from build123d import *

# Parameters (mm, degrees)
F0_R     = 59
F0_R_2   = 49
F1_DEPTH = 3
F0_R_3   = 45
F2_DEPTH = 15
F3_SIZE  = 3


with BuildPart() as f1:
    # F0 (on Top) → F1 (new body)
    with BuildSketch(Plane.XY):
        with Locations((-35.217796, 30.469857)):
            Circle(F0_R)
        with Locations((-35.217796, 30.469857)):
            Circle(F0_R_2, mode=Mode.SUBTRACT)
    extrude(amount=F1_DEPTH)

    # F0 (on Top) → F2 (join)
    with BuildSketch(Plane.XY):
        with Locations((-35.217796, 30.469857)):
            Circle(F0_R_2)
        with Locations((-35.217796, 30.469857)):
            Circle(F0_R_3, mode=Mode.SUBTRACT)
    extrude(amount=F2_DEPTH)

    # F3
    f3_edges = [f1.edges().sort_by_distance(p)[0] for p in [
        (-80.217796, 30.469857, 15),
    ]]
    chamfer(f3_edges, length=F3_SIZE)


solid = f1.part
The model under review builds one solid part; all positions refer to its coordinate system, in mm. A direction names the side the tool comes from. Round coordinates to 2 decimals unless told otherwise and drop trailing zeros. Write each loop counter-clockwise with the first axis right and the second up, starting at its lowest first coordinate (ties: lowest second). Pieces come first, ordered by that corner, then holes. Notation, with made-up numbers: (-2, 5) - (10, 5) arc R29 cw to (10, 41) - close; hole circle Ø9 at (87.25, 22.5). An arc over 180 degrees is marked (long way). One line per item, written item: value. Start each with the question number.
1. Clearance check with flat-ended pins moving along their axes: P1, Ø1, axis at x = -74, z = 9, coming from the +Y side; P2, Ø6, axis at y = 22.5, z = 12, coming from the +X side; P3, Ø8, axis at y = -9.5, z = 2, coming from the +X side. State where each tip first meets the part, or that it passes through.
2. Consider section A-A on z = 13.5. Write out the cut boundary in (x, y).
3. The part is to be moulded in two halves that separate along Y. For faces 1 (the face through (-41.076, 75.087, 5.916)), 2 (the face through (-71.33, 63.59, 8.92)), 3 (the face through (-49, -13, 0)), say which applies: released by +Y, released by -Y, zero draft, split by the parting line, or undercut.
4. Consider section B-B on z = 7. Write out the cut boundary in (x, y), and give its area (3 significant figures).
5. To check wall thickness, follow L1, parallel to Y at x = -11, z = 6.75; L2, parallel to Y at x = -46, z = 2.75; L3, parallel to X at y = 35, z = 10.25. State the ranges of each line that lie inside material, in increasing order. Write a range as from..to.
6. Machinability: for faces 4 (the face through (-48.008, -27.127, 1.479)), 5 (the face through (-27, 79, 3)), which of the approach directions +Z, -Z, +X, -X, +Y, -Y give a long, thin tool a straight path to every point of the face, cutting with its end or side? Answer none if there is none.
Checks:
1. P1: stops at y = 61.06
1. P2: stops at x = 13.53
1. P3: stops at x = 11.55
2. outline: circle Ø98 at (-35.22, 30.47); hole circle Ø93 at (-35.22, 30.47)
3. face 1: undercut
3. face 2: split by the parting line
3. face 3: zero draft
4. outline: circle Ø98 at (-35.22, 30.47); hole circle Ø90 at (-35.22, 30.47)
4. area: 1,180 mm^2
5. L1: y = -12.13..-7.46, 68.4..73.07
5. L2: y = -27.54..-13.22, 74.16..88.48
5. L3: x = -84.01..-79.99, 9.55..13.57
6. face 4: +Z, -Z
6. face 5: +Z
